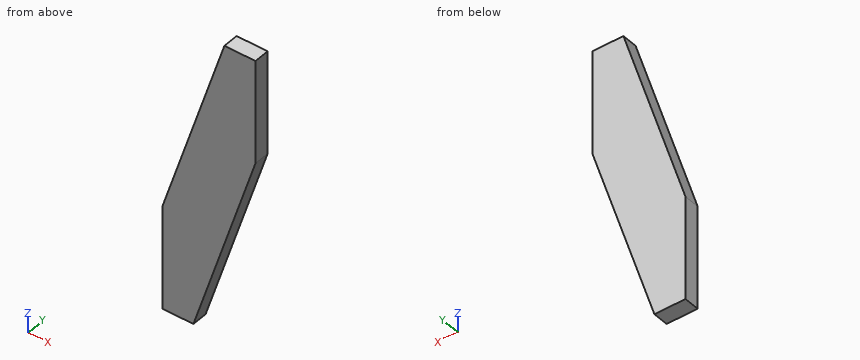
Solid Edge part; units mm, degrees
sketch "Sketch1" plane through (0, 0, 0) normal (0, -1, 0) x (1, 0, 0)
  line L0 (-8.2572, -14.4281) -> (-5.2572, -14.4281)
  line L1 (0.7428, 4.2582) -> (-5.2572, -14.4281)
  line L2 (0.7428, 14.2582) -> (0.7428, 4.2582)
  line L3 (-2.2572, 14.2582) -> (0.7428, 14.2582)
  line L4 (-8.2572, -4.4281) -> (-2.2572, 14.2582)
  line L5 (-8.2572, -14.4281) -> (-8.2572, -4.4281)
  dimension "D1" = 0.7428
extrude "Protrusion1" add sketch "Sketch1" against normal blind 1.5
CAD build for the part. Positions are in the model's coordinates, mm. Coordinates: 2 decimals unless noted, no trailing zeros. Write each loop counter-clockwise with the first axis right and the second up, starting at its lowest first coordinate (ties: lowest second). Pieces come first, ordered by that corner, then holes.
(1) Flat gauge pin, fed straight in: pin 1 (2 mm diameter, centred on x = -0.5, z = -8, fed in from -Y). Where does the tip first touch, or does it go through?
(2) Drill centre lines: probe 1 along X at (y, z) = (1.3, -0.25); probe 2 along X at (y, z) = (0.45, -12). Where is each one in solid material? Low to high.
(3) Cut at A-A, the plane y = 0.75. List the corners of the cut face in (x, z), and give its area (3 significant figures).
(4) Cut at B-B, the plane x = 0. List the corners of the cut face in (y, z), and give its area (3 significant figures).
(5) Cut at C-C, the plane z = -11.75. List the corners of the cut face in (x, y).
Geometry says:
1. pin 1: passes through
2. probe 1: x = -6.92 to -0.7
2. probe 2: x = -8.26 to -4.48
3. outline: (-8.26, -14.43) - (-5.26, -14.43) - (0.74, 4.26) - (0.74, 14.26) - (-2.26, 14.26) - (-8.26, -4.43) - close
3. area: 146 mm2
4. outline: (0, 1.94) - (1.5, 1.94) - (1.5, 14.26) - (0, 14.26) - close
4. area: 18.5 mm2
5. outline: (-8.26, 0) - (-4.4, 0) - (-4.4, 1.5) - (-8.26, 1.5) - close
